For this review, take the finished solid that the model builds, in its own axes (mm). Face numbers are marked on the shaded views. A direction names the side the tool comes from. Give positions to 0.01 mm unless a question says otherwise; leave off trailing zeros. Write each loop counter-clockwise with the first axis right and the second up, starting at its lowest first coordinate (ties: lowest second). Pieces come first, ordered by that corner, then holes.
Q1. We need section C-C (y = -10). Write out the cut boundary in (x, z), then the cut area to 3 significant figures.
Q2. For line 1 (X direction, y = -106, z = 7); line 2 (X direction, y = -9, z = 2.75); line 3 (Y direction, x = -88.5, z = 11.5), list the stretches that pass through material, from the lowest coordinate up.
Q3. We need section A-A (z = 8.25). Write out the cut boundary in (x, y), then the cut area to 3 significant figures.
Q4. Machinability: for the marked faces 1, 2, 3 and 4, which of the approach directions +Z, -Z, +X, -X, +Y, -Y give a long, thin tool a straight path to every point of the face, cutting with its end or side? Answer none if there is none.
Q5. Insertion check: P1, Ø1, axis at x = -6, z = 1, coming from the +Y side; P2, Ø2, axis at y = -10, z = 0.5, coming from the +X side. Each pin has a flat end and moves straight along its axis. Give the tip position at first contact, or say it passes through.
Q6. We need section D-D (x = -162.5). Write out the cut boundary in (y, z).
Q7. We need section B-B (x = -34.5). Write out the cut boundary in (y, z).
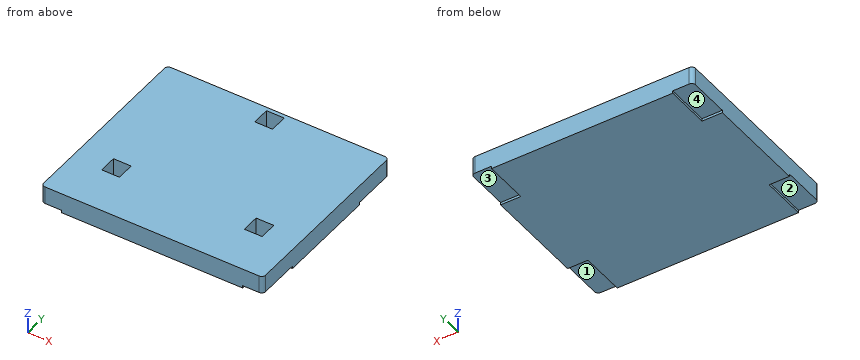
```python
from build123d import *

# Parameters (mm, degrees)
SKETCH1_W           = 175
SKETCH1_H           = 150
BOSS_EXTRUDE1_DEPTH = 16
SKETCH2_W           = 14
SKETCH2_H           = 14
CUT_EXTRUDE1_DEPTH  = 14
SKETCH4_W           = 16
SKETCH4_H           = 35
CUT_EXTRUDE5_DEPTH  = 2
FILLET1_R           = 3


with BuildPart() as part:
    # Sketch1 → Boss-Extrude1 (new body)
    with BuildSketch(Plane.XY):
        with Locations((-87.5, -75)):
            Rectangle(SKETCH1_W, SKETCH1_H)
    extrude(amount=BOSS_EXTRUDE1_DEPTH)

    # Sketch2 → Cut-Extrude1 (cut)
    with BuildSketch(Plane.XY.offset(16)):
        with Locations((-87.5, -10)):
            Rectangle(SKETCH2_W, SKETCH2_H)
        with Locations((-143.791651246, -107.5)):
            Rectangle(SKETCH2_W, SKETCH2_H)
        with Locations((-31.208348754, -107.5)):
            Rectangle(SKETCH2_W, SKETCH2_H)
    extrude(amount=-CUT_EXTRUDE1_DEPTH, mode=Mode.SUBTRACT)

    # Sketch4 → Cut-Extrude5 (cut)
    with BuildSketch(Plane(origin=(0, 0, 0), x_dir=(-1, 0, 0), z_dir=(0, 0, -1))):
        with Locations((167, -17.5)):
            Rectangle(SKETCH4_W, SKETCH4_H)
        with Locations((167, -132.5)):
            Rectangle(SKETCH4_W, SKETCH4_H)
        with Locations((8, -132.5)):
            Rectangle(SKETCH4_W, SKETCH4_H)
        with Locations((8, -17.5)):
            Rectangle(SKETCH4_W, SKETCH4_H)
    extrude(amount=-CUT_EXTRUDE5_DEPTH, mode=Mode.SUBTRACT)

    # Fillet1
    fillet1_edges = [part.edges().sort_by_distance(p)[0] for p in [
        (0, -150, 9),
        (-175, -150, 9),
        (-175, 0, 9),
        (0, 0, 9),
    ]]
    fillet(fillet1_edges, radius=FILLET1_R)


solid = part.part
```
Computed:
1. outline: (-175, 2) - (-159, 2) - (-159, 0) - (-16, 0) - (-16, 2) - (0, 2) - (0, 16) - (-80.5, 16) - (-80.5, 2) - (-94.5, 2) - (-94.5, 16) - (-175, 16) - close
1. area: 2,540 mm2
2. line 1: x = -175 to -150.79, -136.79 to -38.21, -24.21 to 0
2. line 2: x = -175 to -94.5, -80.5 to 0
2. line 3: y = -150 to -17, -3 to 0
3. outline: (-175, -147) arc R3 ccw to (-172, -150) - (-3, -150) arc R3 ccw to (0, -147) - (0, -3) arc R3 ccw to (-3, 0) - (-172, 0) arc R3 ccw to (-175, -3) - close; hole (-150.79, -114.5) - (-136.79, -114.5) - (-136.79, -100.5) - (-150.79, -100.5) - close; hole (-94.5, -17) - (-80.5, -17) - (-80.5, -3) - (-94.5, -3) - close; hole (-38.21, -114.5) - (-24.21, -114.5) - (-24.21, -100.5) - (-38.21, -100.5) - close
3. area: 25,700 mm2
4. face 1: -Z, +X, -Y
4. face 2: -Z, -X, -Y
4. face 3: -Z, +X, +Y
4. face 4: -Z, -X, +Y
5. P1: stops at y = -35
5. P2: stops at x = -16
6. outline: (-150, 2) - (-115, 2) - (-115, 0) - (-35, 0) - (-35, 2) - (0, 2) - (0, 16) - (-150, 16) - close
7. outline: (-150, 0) - (0, 0) - (0, 16) - (-100.5, 16) - (-100.5, 2) - (-114.5, 2) - (-114.5, 16) - (-150, 16) - close
